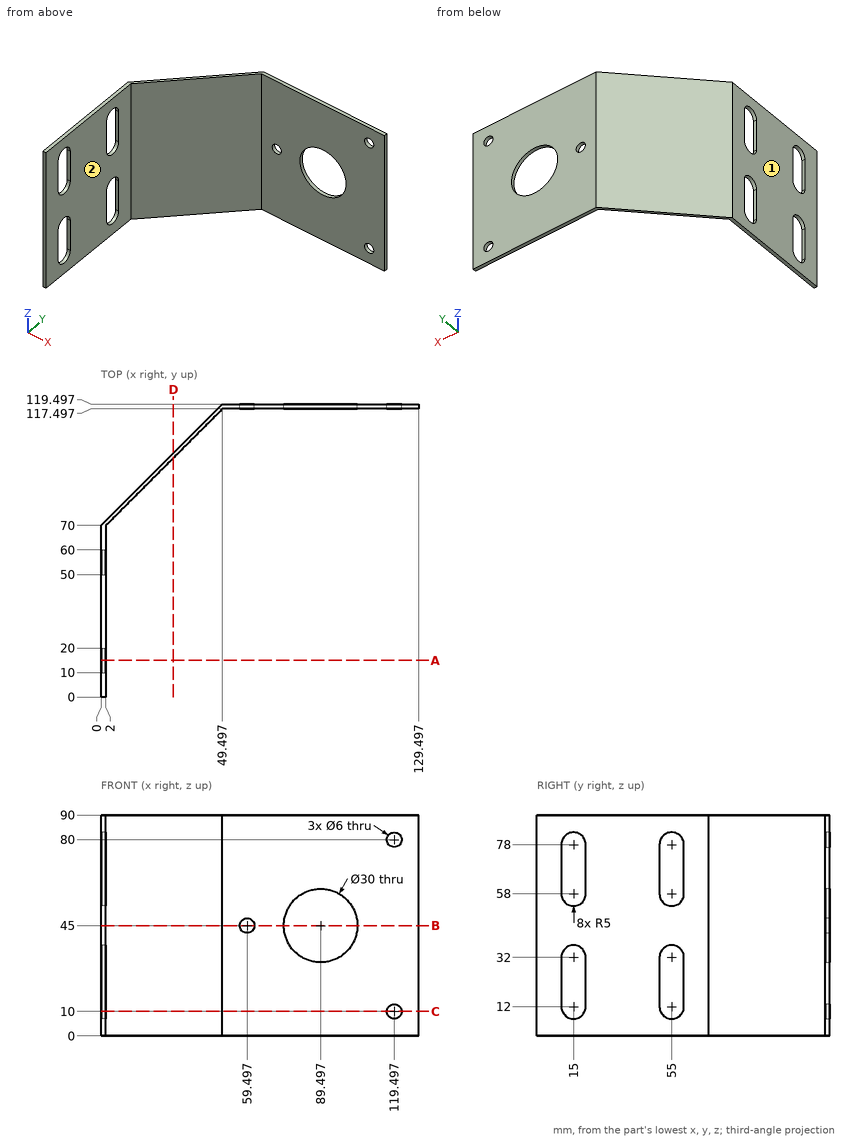
The drawing under review shows one solid part. Ordinate dimensions are in mm from its lowest x, y, z. A direction names the side the tool comes from. Round coordinates to 2 decimals unless told otherwise and drop trailing zeros. Write each loop counter-clockwise with the first axis right and the second up, starting at its lowest first coordinate (ties: lowest second). Pieces come first, ordered by that corner, then holes. Notation, with made-up numbers: (-33, -30.5) -> (-4, -30.5) arc R13 cw to (-4, -8.5) -> close; hole circle Ø5 at (8, 66). An arc over 180 degrees is marked (long way). Put each result on its own line as item: value.
Q1. Machinability: for the marked faces 1 and 2, which of the approach directions +Z, -Z, +X, -X, +Y, -Y give a long, thin tool a straight path to every point of the face, cutting with its end or side? Answer none if there is none.
Determined:
face 1: +Z, -Z, -X, +Y, -Y
face 2: +Z, -Z, +X, -Y
Q2. Consider section C-C on z = 10. State the section outline as (x, y) points.
Determined:
outline: (0, 0) -> (2, 0) -> (2, 10.42) -> (0, 10.42) -> close; (0, 19.58) -> (2, 19.58) -> (2, 50.42) -> (0, 50.42) -> close; (0, 59.58) -> (2, 59.58) -> (2, 70) -> (49.5, 117.5) -> (116.5, 117.5) -> (116.5, 119.5) -> (49.5, 119.5) -> (0, 70) -> close; (122.5, 117.5) -> (129.5, 117.5) -> (129.5, 119.5) -> (122.5, 119.5) -> close
Q3. Clearance check with flat-ended pins moving along their axes: pin 1 Ø1 at (x, z) = (1.5, 68) entering from +Y; pin 2 Ø2 at (y, z) = (97, 59.5) entering from +X; pin 3 Ø0.6 at (x, z) = (1.5, 19) entering from -Y; pin 4 Ø7 at (x, z) = (119.5, 10) entering from -Y. State where each tip first meets the part, or that it passes through.
Determined:
pin 1: stops at y = 72
pin 2: stops at x = 30
pin 3: stops at y = 0
pin 4: stops at y = 117.5
Q4. Consider section B-B on z = 45. State the section outline as (x, y) points, and give its area (3 significant figures).
Determined:
outline: (0, 0) -> (2, 0) -> (2, 70) -> (49.5, 117.5) -> (56.5, 117.5) -> (56.5, 119.5) -> (49.5, 119.5) -> (0, 70) -> close; (62.5, 117.5) -> (74.5, 117.5) -> (74.5, 119.5) -> (62.5, 119.5) -> close; (104.5, 117.5) -> (129.5, 117.5) -> (129.5, 119.5) -> (104.5, 119.5) -> close
area: 325 mm^2
Q5. To check wall thickness, follow L1, parallel to X at y = 118, z = 10 (1 decimal); L2, parallel to Y at x = 79.5, z = 6.5; L3, parallel to X at y = 35, z = 24. State the ranges of each line that lie inside material, in increasing order. Write a range as [from, to].
Determined:
L1: x = [48, 116.5], [122.5, 129.5]
L2: y = [117.5, 119.5]
L3: x = [0, 2]
Q6. Consider section D-D on x = 29.5. State the section outline as (y, z) points, and give its area (3 significant figures).
Determined:
outline: (97.5, 0) -> (99.5, 0) -> (99.5, 90) -> (97.5, 90) -> close
area: 180 mm^2
Q7. Consider section A-A on y = 15. State the section outline as (x, z) points.
Determined:
outline: (0, 0) -> (2, 0) -> (2, 7) -> (0, 7) -> close; (0, 37) -> (2, 37) -> (2, 53) -> (0, 53) -> close; (0, 83) -> (2, 83) -> (2, 90) -> (0, 90) -> close
